Autodesk Inventor part; units mm, degrees
ref_plane "YZ Plane" through (0, 0, 0) normal (1, 0, 0) x (0, 1, 0)
ref_plane "XZ Plane" through (0, 0, 0) normal (0, 1, 0) x (-1, 0, 0)
ref_plane "XY Plane" through (0, 0, 0) normal (0, 0, 1) x (1, 0, 0)
sketch "Sketch1" plane through (0, 0, 0) normal (0, 0, 1) x (1, 0, 0)
  line L0 (0, 0) -> (25.4, 0)
  line L1 (25.4, 0) -> (25.4, 25.4)
  line L2 (25.4, 25.4) -> (0, 25.4)
  line L3 (0, 25.4) -> (0, 0)
  line L4 (3.175, 22.225) -> (22.225, 22.225)
  line L5 (22.225, 22.225) -> (22.225, 3.175)
  line L6 (22.225, 3.175) -> (3.175, 3.175)
  line L7 (3.175, 3.175) -> (3.175, 22.225)
  dimension "d0" = 25.4
  dimension "d1" = 25.4
  dimension "d2" = 3.175
extrude "Extrusion1" add sketch "Sketch1" along normal blind 127
sketch "Sketch2" plane through (25.4, 0, 0) normal (1, 0, 0) x (0, 0, -1)
  line L0 (0, 0) -> (0, 25.4)
  line L1 (-127, 0) -> (-127, 25.4)
  line L2 (0, 0) -> (-127, 0)
  line L3 (-127, 12.7) -> (-114.3, 12.7) construction
  line L4 (0, 12.7) -> (-12.7, 12.7) construction
  circle A0 centre (-114.3, 12.7) radius 3.302
  line L5 (0, 25.4) -> (-127, 25.4)
  line L6 (-114.3, 12.7) -> (-12.7, 12.7) construction
  circle A1 centre (-101.6, 12.7) radius 3.302
  circle A2 centre (-88.9, 12.7) radius 3.302
  circle A3 centre (-76.2, 12.7) radius 3.302
  circle A4 centre (-63.5, 12.7) radius 3.302
  circle A5 centre (-50.8, 12.7) radius 3.302
  circle A6 centre (-38.1, 12.7) radius 3.302
  circle A7 centre (-25.4, 12.7) radius 3.302
  circle A8 centre (-12.7, 12.7) radius 3.302
  dimension "d5" = 12.7
  dimension "d7" = 6.604
  dimension "d13" = 127
  dimension "d16" = 12.7
extrude "Extrusion2" cut sketch "Sketch2" against normal through all contours A0 | A1 | A2 | A3 | A4 | A5 | A6 | A7 | A8
equation "\"d16\" = -0.25 * d5 + 0.125 * d13"
properties part number "Chassis V1.500 Part8" material "Aluminum 6061"
Could you check a few things on this model? Use its own coordinates, in mm. A direction names the side the tool comes from. Give positions to 0.01 mm unless a question says otherwise; leave off trailing zeros. Order: outer loops, then holes, each group sorted by start corner. A loop starts at its lowest first (then second) coordinate and runs counter-clockwise, first axis right, second up. Notation, with made-up numbers: (17.5, -6.75) -> (36.5, -6.75) arc R5 ccw to (36.5, 1.25) -> close; hole circle Ø1 at (-28, -28.75). An arc over 180 degrees is marked (long way). Answer in a Markdown table with one row per item. Add a question column.
Item 1: We'd pull the mould along X, two halves only. Please class faces 3 (the flat face through (25.4, 7, 63)), 4 (the flat face through (22.225, 9, 63)), 5 (the cylindrical face through (1.61, 13.69, 111.15)): pulls with the +X half, pulls with the -X half, needs draft (parallel to the pull), parting line crosses it, or undercut.
Item 2: For faces 1 (the flat face through (13, 22.225, 63)), 2 (the flat face through (24, 13, 127)), which set-ups out of +Z, -Z, +X, -X, +Y, -Y let a thin tool reach every point of the face, with its end or its side?
Item 3: Imagine slicing it at D-D (z = 63). List the corners of the cut face in (x, y) for me (3 decimals).
Item 4: Please list where these lines run through material, in increasing order: probe 1 along X at (y, z) = (11, 21.5) (3 decimals); probe 2 along Y at (x, z) = (23.1, 38.1).
Item 5: Imagine slicing it at B-B (z = 88.9). List the corners of the cut face in (x, y) for me (3 decimals), and give its area (3 significant figures).
Item 6: Imagine slicing it at A-A (y = 7). List the corners of the cut face in (x, z) for me (3 decimals).
Result:
| question | item | result |
|---|---|---|
| 1 | face 3 | pulls with the +X half |
| 1 | face 4 | undercut |
| 1 | face 5 | needs draft |
| 2 | face 1 | +Z, -Z |
| 2 | face 2 | +Z, +X, -X, +Y, -Y |
| 3 | outline | (0, 0) -> (25.4, 0) -> (25.4, 9.436) -> (22.225, 9.436) -> (22.225, 3.175) -> (3.175, 3.175) -> (3.175, 9.436) -> (0, 9.436) -> close; (0, 15.964) -> (3.175, 15.964) -> (3.175, 22.225) -> (22.225, 22.225) -> (22.225, 15.964) -> (25.4, 15.964) -> (25.4, 25.4) -> (0, 25.4) -> close |
| 4 | probe 1 | 0 to 3.175, 22.225 to 25.4 |
| 4 | probe 2 | 0 to 9.4, 16 to 25.4 |
| 5 | outline | (0, 0) -> (25.4, 0) -> (25.4, 9.398) -> (22.225, 9.398) -> (22.225, 3.175) -> (3.175, 3.175) -> (3.175, 9.398) -> (0, 9.398) -> close; (0, 16.002) -> (3.175, 16.002) -> (3.175, 22.225) -> (22.225, 22.225) -> (22.225, 16.002) -> (25.4, 16.002) -> (25.4, 25.4) -> (0, 25.4) -> close |
| 5 | area | 240 mm2 |
| 6 | outline | (0, 0) -> (3.175, 0) -> (3.175, 127) -> (0, 127) -> close; (22.225, 0) -> (25.4, 0) -> (25.4, 127) -> (22.225, 127) -> close |
